from build123d import *

# Parameters (mm, degrees)
F0_W     = 762
F0_H     = 101.6
F0_R     = 12.7
F2_DEPTH = 6.35
F3_SIZE  = 6.35
F4_W     = 9.525
F4_H     = 50.8
F5_DEPTH = 6.351
F6_R     = 1.6002


with BuildPart() as f2:
    # F0 (on Front) → F2 (new body)
    with BuildSketch(Plane.XZ):
        with Locations((218.576816025, -2.0831003785)):
            Rectangle(F0_W, F0_H)
        with Locations((-98.923183975, -2.0831003785)):
            Circle(F0_R, mode=Mode.SUBTRACT)
        with Locations((28.076816025, -2.0831003785)):
            Circle(F0_R, mode=Mode.SUBTRACT)
        with Locations((155.076816025, -2.0831003785)):
            Circle(F0_R, mode=Mode.SUBTRACT)
        with Locations((282.076816025, -2.0831003785)):
            Circle(F0_R, mode=Mode.SUBTRACT)
        with Locations((409.076816025, 0.1906121615)):
            Circle(F0_R, mode=Mode.SUBTRACT)
        with Locations((536.076816025, 0.1906121615)):
            Circle(F0_R, mode=Mode.SUBTRACT)
    extrude(amount=F2_DEPTH)

    # F3
    f3_edges = [f2.edges().sort_by_distance(p)[0] for p in [
        (-162.423184, -3.175, 48.7169),
        (-162.423184, -3.175, -52.8831),
        (599.576816, -3.175, -52.8831),
        (599.576816, -3.175, 48.7169),
    ]]
    chamfer(f3_edges, length=F3_SIZE)

    # F4 (on face) → F5 (cut, through all)
    with BuildSketch(Plane.XZ.offset(6.35)):
        with Locations((-63.985483975, -2.0831003785)):
            Rectangle(F4_W, F4_H)
        with Locations((-51.285483975, -2.0831003785)):
            Rectangle(F4_W, F4_H)
        with Locations((-38.585483975, -2.0831003785)):
            Rectangle(F4_W, F4_H)
        with Locations((-25.885483975, -2.0831003785)):
            Rectangle(F4_W, F4_H)
        with Locations((-13.185483975, -2.0831003785)):
            Rectangle(F4_W, F4_H)
        with Locations((63.014516025, -2.0831003785)):
            Rectangle(F4_W, F4_H)
        with Locations((75.714516025, -2.0831003785)):
            Rectangle(F4_W, F4_H)
        with Locations((88.414516025, -2.0831003785)):
            Rectangle(F4_W, F4_H)
        with Locations((101.114516025, -2.0831003785)):
            Rectangle(F4_W, F4_H)
        with Locations((113.814516025, -2.0831003785)):
            Rectangle(F4_W, F4_H)
        with Locations((190.014516025, -2.0831003785)):
            Rectangle(F4_W, F4_H)
        with Locations((202.714516025, -2.0831003785)):
            Rectangle(F4_W, F4_H)
        with Locations((215.414516025, -2.0831003785)):
            Rectangle(F4_W, F4_H)
        with Locations((228.114516025, -2.0831003785)):
            Rectangle(F4_W, F4_H)
        with Locations((240.814516025, -2.0831003785)):
            Rectangle(F4_W, F4_H)
        with Locations((317.014516025, -2.0831003785)):
            Rectangle(F4_W, F4_H)
        with Locations((329.714516025, -2.0831003785)):
            Rectangle(F4_W, F4_H)
        with Locations((342.414516025, -2.0831003785)):
            Rectangle(F4_W, F4_H)
        with Locations((355.114516025, -2.0831003785)):
            Rectangle(F4_W, F4_H)
        with Locations((367.814516025, -2.0831003785)):
            Rectangle(F4_W, F4_H)
        with Locations((444.014516025, -2.0831003785)):
            Rectangle(F4_W, F4_H)
        with Locations((456.714516025, -2.0831003785)):
            Rectangle(F4_W, F4_H)
        with Locations((469.414516025, -2.0831003785)):
            Rectangle(F4_W, F4_H)
        with Locations((482.114516025, -2.0831003785)):
            Rectangle(F4_W, F4_H)
        with Locations((494.814516025, -2.0831003785)):
            Rectangle(F4_W, F4_H)
    extrude(amount=-F5_DEPTH, mode=Mode.SUBTRACT)

    # F6
    f6_edges = [f2.edges().sort_by_distance(p)[0] for p in [
        (218.576816, -6.35, 48.7169),
        (-162.423184, 0, -2.0831),
        (-159.248184, -6.35, 45.5419),
        (-162.423184, -6.35, -2.0831),
        (-159.248184, -6.35, -49.7081),
        (218.576816, -6.35, -52.8831),
        (596.401816, -6.35, -49.7081),
        (599.576816, -6.35, -2.0831),
        (596.401816, -6.35, 45.5419),
        (596.401816, 0, 45.5419),
        (218.576816, 0, 48.7169),
        (599.576816, 0, -2.0831),
        (596.401816, 0, -49.7081),
        (218.576816, 0, -52.8831),
        (-159.248184, 0, -49.7081),
    ]]
    fillet(f6_edges, radius=F6_R)


solid = f2.part
Input: part model. Units: mm. Frame: model coordinates. Coordinates: 2 decimals unless noted, no trailing zeros.
Q1. Material intervals for line 1 (Z direction, x = 213.5, y = -4.25); line 2 (Z direction, x = 88, y = -5.5); line 3 (Z direction, x = 179, y = -1), sorted ascending.
Q2. Contact query for a flat-ended pin moving along its axis: pin 1 (1.9 mm diameter, centred on y = -1.5, z = -11, fed in from +X). Output: stop coordinate, or through.
Q3. Draft query along Z for faces 1 (the face through (526.716, -3.131, 8.774)), 2 (the face through (213, 0, 31)). Return one class per face: +Z half, -Z half, draft (parallel to the pull), parting line (faces both ways), or undercut.
Q4. Cut plane A-A (z = -21). Give the number of separate pieces and of enclosed holes in the cut face, then the cut area to 3 significant figures.
Working result:
1. line 1: z = -52.88 to -27.48, 23.32 to 48.72
1. line 2: z = -52.7 to -27.48, 23.32 to 48.53
1. line 3: z = -52.77 to 48.6
2. pin 1: stops at x = 599.58
3. face 1: undercut
3. face 2: draft
4. separate pieces: 26
4. enclosed holes: 0
4. area: 3,320 mm2
